Geometry check sheet. Reference: the model listing, model coordinates, mm. Face numbers are marked on the shaded views. Round coordinates to 2 decimals unless told otherwise and drop trailing zeros. Write each loop counter-clockwise with the first axis right and the second up, starting at its lowest first coordinate (ties: lowest second). Pieces come first, ordered by that corner, then holes.
Item 1: Cross-section at B-B (y = 2.25). Enter the section's corners in (x, z).
Item 2: Draft check along Z on the marked faces 1, 2 and 3. Enter one of: pulls with the +Z half, pulls with the -Z half, needs draft (parallel to the pull), parting line crosses it, or undercut.
Item 3: Cross-section at A-A (x = 0). Enter the section's corners in (y, z), then the cut area to 3 significant figures.
Item 4: Cross-section at C-C (z = 0). Enter the section's corners in (x, y), then the cut area to 3 significant figures.
Item 5: Scan lines: probe 1 along X at (y, z) = (7.75, 0); probe 2 along Y at (x, z) = (-6.75, -6); probe 3 along X at (y, z) = (6.5, 2.75). Record each from-to range of solid material in increasing order.
Item 6: Depth check by flat-ended pin: P1, Ø1, axis at x = 2, z = 7.5, coming from the -Y side; P2, Ø5, axis at y = 6.5, z = 8.5, coming from the -X side; P3, Ø1.5, axis at x = 3.5, z = 12, coming from the +Y side. Enter the tip coordinate at first touch or a pass-through.
from build123d import *

# Parameters (mm, degrees)
SKETCH1_R                = 12.7
BOSS_EXTRUDE1_DEPTH      = 12.7
FILLET1_R                = 2.54
SHELL1_T                 = -1.27
BOSS_EXTRUDE2_REACH      = 36.29
BOSS_EXTRUDE2_END_RADIUS = 12.7
SKETCH4_W                = 7.62
SKETCH4_H                = 1.651
FILLET2_R                = 2.54


with BuildPart() as part:
    # Sketch1 → Boss-Extrude1 (new body)
    with BuildSketch(Plane(origin=(0, 0, 0), x_dir=(1, 0, 0), z_dir=(0, 1, 0))):
        with Locations(Location((0, 0, 0), (0, 0, 90))):
            Circle(SKETCH1_R)
    extrude(amount=BOSS_EXTRUDE1_DEPTH)

    # Fillet1
    fillet1_edges = [part.edges().sort_by_distance(p)[0] for p in [
        (0, 12.7, 12.7),
    ]]
    fillet(fillet1_edges, radius=FILLET1_R)

    # Shell1
    shell1_openings = [part.faces().sort_by_distance(p)[0] for p in [
        (0, 0, 0),
    ]]
    offset(amount=SHELL1_T, openings=shell1_openings, kind=Kind.INTERSECTION)

    # Boss-Extrude2: up to this cylinder (the profile starts outside it)
    boss_extrude2_end = Plane(origin=(0, 0.8255, 0), z_dir=(0, -1, 0)) * Cylinder(BOSS_EXTRUDE2_END_RADIUS, 98.98, mode=Mode.PRIVATE)
    # Sketch4 → Boss-Extrude2 (add, up to the surface)
    with BuildSketch(Plane.XY.offset(16.51), mode=Mode.PRIVATE) as boss_extrude2_sk1:
        with Locations((0, 0.8255)):
            Rectangle(SKETCH4_W, SKETCH4_H)
    boss_extrude2_tool1 = extrude(boss_extrude2_sk1.sketch, amount=-BOSS_EXTRUDE2_REACH, mode=Mode.PRIVATE) - boss_extrude2_end
    add(boss_extrude2_tool1.solids().sort_by_distance((0, 0.8255, 16.51))[0])

    # Fillet2
    fillet2_edges = [part.edges().sort_by_distance(p)[0] for p in [
        (-3.81, 0.8255, 16.51),
        (3.81, 0.8255, 16.51),
    ]]
    fillet(fillet2_edges, radius=FILLET2_R)


solid = part.part
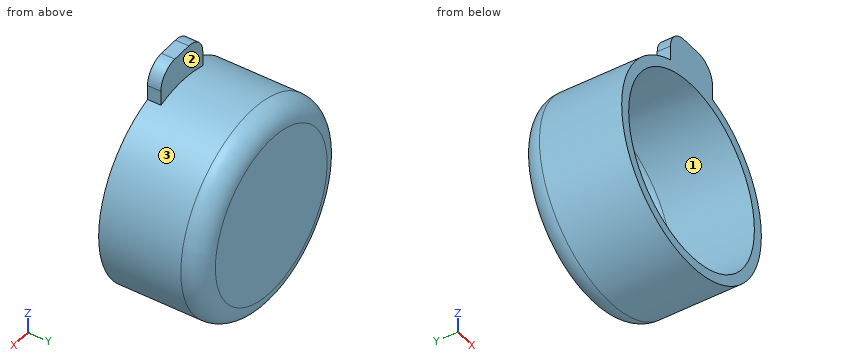
Resolved:
1. outline: circle Ø25.4 at (0, 0); hole circle Ø22.86 at (0, 0)
2. face 1: undercut
2. face 2: needs draft
2. face 3: parting line crosses it
3. outline: (0, -12.7) - (10.16, -12.7) arc R2.54 ccw to (12.7, -10.16) - (12.7, 10.16) arc R2.54 ccw to (10.16, 12.7) - (1.65, 12.7) - (1.65, 16.51) - (0, 16.51) - (0, 11.43) - (10.16, 11.43) arc R1.27 cw to (11.43, 10.16) - (11.43, -10.16) arc R1.27 cw to (10.16, -11.43) - (0, -11.43) - close
3. area: 65.5 mm2
4. outline: (-12.7, 0) - (-11.43, 0) - (-11.43, 10.16) arc R1.27 cw to (-10.16, 11.43) - (10.16, 11.43) arc R1.27 cw to (11.43, 10.16) - (11.43, 0) - (12.7, 0) - (12.7, 10.16) arc R2.54 ccw to (10.16, 12.7) - (-10.16, 12.7) arc R2.54 ccw to (-12.7, 10.16) - close
4. area: 59.2 mm2
5. probe 1: x = -12.7 to -11.43, 11.43 to 12.7
5. probe 2: y = 11.43 to 12.7
5. probe 3: x = -12.4 to -11.09, 11.09 to 12.4
6. P1: stops at y = 11.43
6. P2: stops at x = -11.19
6. P3: stops at y = 12.14
